Design review of the part built by this model. Coordinates are the model's own, in mm. Face numbers are marked on the shaded views. A direction names the side the tool comes from. Coordinates: 2 decimals unless noted, no trailing zeros. Order: outer loops, then holes, each group sorted by start corner. A loop starts at its lowest first (then second) coordinate and runs counter-clockwise, first axis right, second up. Notation, with made-up numbers: M 22,-7 L 76,-7 A11 ccw 76,0 Z; hole C 72,67.5 d5. An arc over 180 degrees is marked long. Answer in a Markdown table with one row per item.
from build123d import *

# Parameters (mm, degrees)
SKETCH1_W           = 100
SKETCH1_H           = 100
SKETCH1_R           = 1.75
BOSS_EXTRUDE1_DEPTH = 10
BOSS_EXTRUDE2_DEPTH = 4


with BuildPart() as part:
    # Sketch1 → Boss-Extrude1 (new body)
    with BuildSketch(Plane.XY):
        with Locations((-126.253776435, 13.202416918)):
            Rectangle(SKETCH1_W, SKETCH1_H)
        with Locations((-156.253776435, -31.797583082)):
            Circle(SKETCH1_R, mode=Mode.SUBTRACT)
        with Locations((-96.253776435, -31.797583082)):
            Circle(SKETCH1_R, mode=Mode.SUBTRACT)
    extrude(amount=BOSS_EXTRUDE1_DEPTH)

    # Sketch2 → Boss-Extrude2 (add, symmetric)
    with BuildSketch(Plane(origin=(0, 13.202416918, 0), x_dir=(1, 0, 0), z_dir=(0, 1, 0))):
        with BuildLine():
            ThreePointArc((-76.253776435, 0), (-97.691099578, 5.937794762), (-113.018482317, 22.058823529))
            ThreePointArc((-113.018482317, 22.058823529), (-126.253776435, 30), (-139.489070553, 22.058823529))
            ThreePointArc((-139.489070553, 22.058823529), (-154.816453292, 5.937794762), (-176.253776435, 0))
            Line((-176.253776435, 0), (-76.253776435, 0))
        make_face()
        with BuildLine():
            Line((-131.753776435, 24.526279442), (-126.253776435, 27.701705922))
            Line((-126.253776435, 27.701705922), (-120.753776435, 24.526279442))
            ThreePointArc((-120.753776435, 24.526279442), (-126.253776435, 4), (-131.753776435, 24.526279442))
        make_face(mode=Mode.SUBTRACT)
    extrude(amount=BOSS_EXTRUDE2_DEPTH, both=True)


solid = part.part
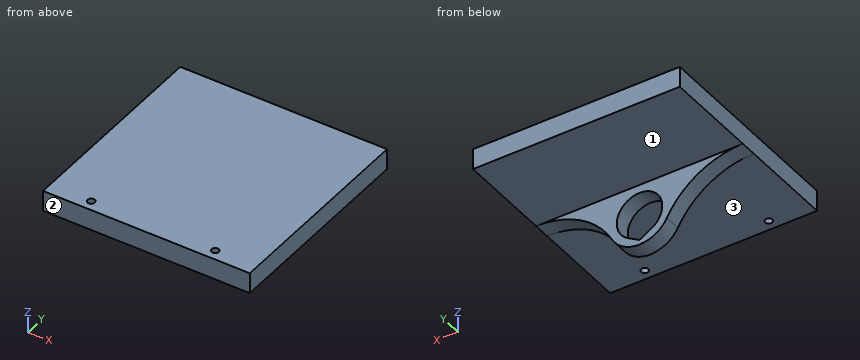
(1) Add section B-B, the plane x = -83.5. Give the boundary of the cut face in (y, z).
Return value:
| item | result |
|---|---|
| outline | M -36.8,0 L 9.2,0 L 9.2,-0.63 L 17.2,-0.63 L 17.2,0 L 63.2,0 L 63.2,10 L -36.8,10 Z |
(2) Insertion check: pin 1 Ø20 at (x, z) = (-126.25, -15) entering from -Y; pin 2 Ø1 at (x, z) = (-140, -8.5) entering from -Y; pin 3 Ø10 at (x, y) = (-111, 24.5) entering from -Z; pin 4 Ø12 at (x, z) = (-136, -21.5) entering from +Y. Each pin has a flat end and moves straight along its axis. Give the tip position at first contact, or say it passes through.
Return value:
| item | result |
|---|---|
| pin 1 | passes through |
| pin 2 | stops at y = 9.2 |
| pin 3 | stops at z = 0 |
| pin 4 | stops at y = 17.2 |
(3) Add section D-D, the plane x = -169.5. Give the boundary of the cut face in (y, z), and give its area (3 significant figures).
Return value:
| item | result |
|---|---|
| outline | M -36.8,0 L 9.2,0 L 9.2,-0.55 L 17.2,-0.55 L 17.2,0 L 63.2,0 L 63.2,10 L -36.8,10 Z |
| area | 1,000 mm2 |
(4) Add section A-A, the plane z = -15. Give the boundary of the cut face in (x, y), and give its area (3 significant figures).
Return value:
| item | result |
|---|---|
| outline | M -144.24,9.2 L -137.25,9.2 L -137.25,17.2 L -144.24,17.2 Z; M -115.25,9.2 L -108.27,9.2 L -108.27,17.2 L -115.25,17.2 Z |
| area | 112 mm2 |
(5) For the marked faces 1, 2 and 3, list the 3-axis set-ups (+Z, -Z, +X, -X, +Y, -Y) from which the entire face can be reached by the end or side of a thin tool; tool diameter is ignored.
Return value:
| item | result |
|---|---|
| face 1 | -Z, +X, -X, +Y |
| face 2 | +Z, -Z, +X, -X, -Y |
| face 3 | -Z, +X, -X, -Y |
(6) Add section C-C, the plane y = 5. Give the boundary of the cut face in (x, z), and give its area (3 significant figures).
Return value:
| item | result |
|---|---|
| outline | M -176.25,0 L -76.25,0 L -76.25,10 L -176.25,10 Z |
| area | 1,000 mm2 |
(7) For line 1 along Z through (x, y) = (-100, -23); line 2 along X through (y, z) = (13, -15); line 3 along Y through (x, z) = (-113.5, -1.5), list the stretches that pass through material, from the lowest coordinate up. Write a range as from..to.
Return value:
| item | result |
|---|---|
| line 1 | z = 0..10 |
| line 2 | x = -144.24..-137.25, -115.25..-108.27 |
| line 3 | y = 9.2..17.2 |
